The listing builds one solid part. Answer for the finished solid, in the listing's coordinates (mm). A direction names the side the tool comes from. Coordinates: 2 decimals unless noted, no trailing zeros. Return JSON: item names as keys, results as strings. Group by question number.
1. Straight lines are drawn through the part: L1, parallel to X at y = 0.25, z = 4; L2, parallel to X at y = 0.4, z = 0; L3, parallel to Z at x = 0, y = 0.4. For each, find the intervals that lie inside material, in ascending order. Write a range as from..to.
2. The mould has two halves that part along Z. Classify faces 4 (the face through (0.1, 0.6, -3.1)), 5 (the face through (-16.973, 3.24, -0.343)), 6 (the face through (0, 2, 24.5)): pulls with the +Z half, pulls with the -Z half, needs draft (parallel to the pull), parting line crosses it, or undercut.
3. Given P1, Ø0.7, axis at x = -0.5, z = 3.5, coming from the -Y side; P2, Ø1.7, axis at x = -1, z = 1, coming from the -Y side, each flat-ended and moving along its own axis, determine where each tip first touches the part or whether it passes through.
4. Which of the six approach directions +Z, -Z, +X, -X, +Y, -Y give full straight-line access (tool end or side, diameter ignored) to faces 1 (the face through (13.447, 3.24, -0.343)), 2 (the face through (-29.25, 1, 0)), 3 (the face through (-1.75, 1, 4))?
```python
from build123d import *

# Parameters (mm, degrees)
SKETCH1_W           = 58.5
SKETCH1_H           = 49
SKETCH1_R           = 3.1
BOSS_EXTRUDE1_DEPTH = 1.5
BOSS_EXTRUDE2_DEPTH = 49
CUT_EXTRUDE1_DEPTH  = 1
CHAMFER2_SIZE       = 0.2
CUT_EXTRUDE3_DEPTH  = 64.549193543
BOSS_EXTRUDE3_START = 0.5
SKETCH5_R           = 3.1
BOSS_EXTRUDE3_DEPTH = 0.5
SKETCH6_W           = 3.5
SKETCH6_H           = 2.441191684
CUT_EXTRUDE4_DEPTH  = 0.5
CHAMFER3_SIZE       = 1.5


with BuildPart() as part:
    # Sketch1 → Boss-Extrude1 (new body)
    with BuildSketch(Plane(origin=(0, 0, 0), x_dir=(1, 0, 0), z_dir=(0, 1, 0))):
        Rectangle(SKETCH1_W, SKETCH1_H)
        with Locations(Location((0, 0, 0), (0, 0, 270))):
            Circle(SKETCH1_R, mode=Mode.SUBTRACT)
    extrude(amount=BOSS_EXTRUDE1_DEPTH)

    # Sketch2 → Boss-Extrude2 (add)
    with BuildSketch(Plane(origin=(0, 0, -24.5), x_dir=(-1, 0, 0), z_dir=(0, 0, -1))):
        Polygon((-29.25, 1.5), (29.25, 1.5), (29.25, 2.5), (28.08, 4), (26.91, 2.5), (25.74, 4), (24.57, 2.5), (23.4, 4), (22.23, 2.5), (21.06, 4), (19.89, 2.5), (18.72, 4), (17.55, 2.5), (16.38, 4), (15.21, 2.5), (14.04, 4), (12.87, 2.5), (11.7, 4), (10.53, 2.5), (9.36, 4), (8.19, 2.5), (7.02, 4), (5.85, 2.5), (4.68, 4), (3.51, 2.5), (2.34, 4), (1.17, 2.5), (0, 4), (-1.17, 2.5), (-2.34, 4), (-3.51, 2.5), (-4.68, 4), (-5.85, 2.5), (-7.02, 4), (-8.19, 2.5), (-9.36, 4), (-10.53, 2.5), (-11.7, 4), (-12.87, 2.5), (-14.04, 4), (-15.21, 2.5), (-16.38, 4), (-17.55, 2.5), (-18.72, 4), (-19.89, 2.5), (-21.06, 4), (-22.23, 2.5), (-23.4, 4), (-24.57, 2.5), (-25.74, 4), (-26.91, 2.5), (-28.08, 4), (-29.25, 2.5), align=None)
    extrude(amount=-BOSS_EXTRUDE2_DEPTH)

    # Sketch3 → Cut-Extrude1 (cut)
    with BuildSketch(Plane(origin=(0, 0, 0), x_dir=(-1, 0, 0), z_dir=(0, -1, 0))):
        with BuildLine():
            Line((-1.75, -2.558808316), (-1.75, -5))
            Line((-1.75, -5), (1.75, -5))
            Line((1.75, -5), (1.75, -2.558808316))
            ThreePointArc((1.75, -2.558808316), (0, 3.1), (-1.75, -2.558808316))
        make_face()
    extrude(amount=-CUT_EXTRUDE1_DEPTH, mode=Mode.SUBTRACT)

    # Chamfer2
    chamfer2_edges = [part.edges().sort_by_distance(p)[0] for p in [
        (0, 0, -3.1),
    ]]
    chamfer(chamfer2_edges, length=CHAMFER2_SIZE)

    # Sketch4 → Cut-Extrude3 (cut, through all)
    with BuildSketch(Plane(origin=(29.25, 0, 0), x_dir=(0, 0, -1), z_dir=(1, 0, 0))):
        with BuildLine():
            Line((-23.75, 4), (-24.5, 4))
            Line((-24.5, 4), (-24.5, 3.25))
            ThreePointArc((-24.5, 3.25), (-24.280330086, 3.780330086), (-23.75, 4))
        make_face()
    cut_extrude3 = extrude(amount=-CUT_EXTRUDE3_DEPTH, mode=Mode.SUBTRACT)

    # Mirror1: Cut-Extrude3 across plane
    add(cut_extrude3.mirror(Plane.XY), mode=Mode.SUBTRACT)

    # Sketch5 → Boss-Extrude3 (add)
    with BuildSketch(Plane.XZ.offset(-1.5).offset(BOSS_EXTRUDE3_START)):
        Circle(SKETCH5_R)
    extrude(amount=-BOSS_EXTRUDE3_DEPTH)

    # Sketch6 → Cut-Extrude4 (cut)
    with BuildSketch(Plane.XZ.offset(-1)):
        with Locations((0, 3.779404158)):
            Rectangle(SKETCH6_W, SKETCH6_H)
    extrude(amount=-CUT_EXTRUDE4_DEPTH, mode=Mode.SUBTRACT)

    # Chamfer3
    chamfer3_edges = [part.edges().sort_by_distance(p)[0] for p in [
        (0, 0, 5),
    ]]
    chamfer(chamfer3_edges, length=CHAMFER3_SIZE - 0.0001)  # a hair under: the kernel refuses the full size


solid = part.part
```
Worked out:
{
 "1": {"L1": "-29.25..-1.75, 1.75..29.25", "L2": "-29.25..-3.1, 3.1..29.25", "L3": "-24.5..-3.1, 6.1..24.5"},
 "2": {"face 4": "undercut", "face 5": "needs draft", "face 6": "pulls with the +Z half"},
 "3": {"P1": "y = 1.5", "P2": "y = 1"},
 "4": {"face 1": "+Z, -Z, +Y", "face 2": "+Z, -Z, -X, +Y, -Y", "face 3": "-Y"}
}
